Source: CAD feature listing. Evaluate the final solid. Frame: model axes, mm. A direction names the side the tool comes from. Round coordinates to 2 decimals unless told otherwise and drop trailing zeros. Write each loop counter-clockwise with the first axis right and the second up, starting at its lowest first coordinate (ties: lowest second). Pieces come first, ordered by that corner, then holes. Notation, with made-up numbers: M 6.25,71 L 21.25,71 A13 cw 21.25,76 Z; hole C 24,68 d8. An arc over 180 degrees is marked long. Answer in a Markdown table with one row per item. Add a question column.
Item 1: Cut plane D-D on x = 17. Return loops of the section in (y, z).
Item 2: Mould query, pull axis X, two halves, no side actions, for faces 4 (the face through (-27.542, -1.14, 0.986)), 5 (the face through (-30, -0.118, 1)), 6 (the face through (18.06, 4.9, 0.99)), 7 (the face through (-27.54, 1.93, 0.99)). Classes: released by +X, released by -X, zero draft, split by the parting line, or undercut.
Item 3: Cut plane A-A on x = 10.5. Return loops of the section in (y, z), and give its area (3 significant figures).
Item 4: Cut plane B-B on z = 1.55. Return loops of the section in (x, y).
Item 5: Contact query for flat-ended pins moving along their axis: pin 1 (1 mm diameter, centred on y = 14, z = 1, fed in from +X); pin 2 (1.8 mm diameter, centred on x = -26.54, y = 1.88, fed in from -Z); pin 3 (1 mm diameter, centred on x = -29.5, z = 1, fed in from -Y); pin 4 (0.6 mm diameter, centred on x = -29, z = 1.5, fed in from +Y). Output: stop coordinate, or through.
Item 6: Material intervals for probe 1 along X at (y, z) = (7.5, 1.45); probe 2 along X at (y, z) = (13, 1.8); probe 3 along Y at (x, z) = (-5, 1.1), sorted ascending.
Item 7: Cut plane C-C on y = -9. Return loops of the section in (x, z), and give its area (3 significant figures).
Item 8: Set-up query: faces 1 (the face through (20, 3.882, 1)), 2 (the face through (-28.542, 12, 1)), 3 (the face through (-28.542, -8, 1)). Return all of +Z, -Z, +X, -X, +Y, -Y with unobstructed straight access to the full face (end or side cutting, diameter ignored); none if empty.
from build123d import *

# Parameters (mm, degrees)
SKETCH_1_R      = 1.25
SKETCH_1_R_2    = 1
EXTRUDE_2_DEPTH = 2


with BuildPart() as part:
    # 草圖1 → 填料-伸長2 (new body)
    with BuildSketch(Plane.XY):
        with BuildLine():
            Line((18.058094933, -13.1179941), (-27.541905067, -13.1179941))
            Line((-27.541905067, -13.1179941), (-28.541905067, -13.1179941))
            Line((-28.541905067, -13.1179941), (-28.541905067, -12.1179941))
            Line((-28.541905067, -12.1179941), (-28.541905067, -2.1179941))
            ThreePointArc((-28.541905067, -2.1179941), (-27.541905067, -1.1179941), (-28.541905067, -0.1179941))
            Line((-28.541905067, -0.1179941), (-30.541905067, -0.1179941))
            Line((-30.541905067, -0.1179941), (-30.541905067, 3.8820059))
            Line((-30.541905067, 3.8820059), (-28.541905067, 3.8820059))
            ThreePointArc((-28.541905067, 3.8820059), (-27.541905067, 4.8820059), (-28.541905067, 5.8820059))
            Line((-28.541905067, 5.8820059), (-28.541905067, 9.8820059))
            Line((-28.541905067, 9.8820059), (-28.541905067, 10.8820059))
            Line((-28.541905067, 10.8820059), (-28.541905067, 16.8820059))
            Line((-28.541905067, 16.8820059), (-28.541905067, 17.8820059))
            Line((-28.541905067, 17.8820059), (-27.541905067, 17.8820059))
            Line((-27.541905067, 17.8820059), (18.058094933, 17.8820059))
            Line((18.058094933, 17.8820059), (19.058094933, 17.8820059))
            Line((19.058094933, 17.8820059), (19.058094933, 16.8820059))
            Line((19.058094933, 16.8820059), (19.058094933, 10.8820059))
            Line((19.058094933, 10.8820059), (19.058094933, 9.8820059))
            Line((19.058094933, 9.8820059), (19.058094933, 5.8820059))
            ThreePointArc((19.058094933, 5.8820059), (18.058094933, 4.8820059), (19.058094933, 3.8820059))
            Line((19.058094933, 3.8820059), (21.058094933, 3.8820059))
            Line((21.058094933, 3.8820059), (21.058094933, -0.1179941))
            Line((21.058094933, -0.1179941), (19.058094933, -0.1179941))
            ThreePointArc((19.058094933, -0.1179941), (18.058094933, -1.1179941), (19.058094933, -2.1179941))
            Line((19.058094933, -2.1179941), (19.058094933, -12.1179941))
            Line((19.058094933, -12.1179941), (19.058094933, -13.1179941))
            Line((19.058094933, -13.1179941), (18.058094933, -13.1179941))
        make_face()
        with Locations((11.058094933, -5.1179941)):
            Circle(SKETCH_1_R, mode=Mode.SUBTRACT)
        with Locations((-26.541905067, 1.8820059)):
            Circle(SKETCH_1_R_2, mode=Mode.SUBTRACT)
        with Locations((17.058094933, 1.8820059)):
            Circle(SKETCH_1_R_2, mode=Mode.SUBTRACT)
        with Locations((-4.741905067, 13.8820059)):
            Circle(SKETCH_1_R_2, mode=Mode.SUBTRACT)
    extrude(amount=EXTRUDE_2_DEPTH)


solid = part.part
Results below:
| question | item | result |
|---|---|---|
| 1 | outline | M -13.12,0 L 0.88,0 L 0.88,2 L -13.12,2 Z; M 2.88,0 L 17.88,0 L 17.88,2 L 2.88,2 Z |
| 2 | face 4 | released by -X |
| 2 | face 5 | zero draft |
| 2 | face 6 | released by +X |
| 2 | face 7 | undercut |
| 3 | outline | M -13.12,0 L -6.24,0 L -6.24,2 L -13.12,2 Z; M -4,0 L 17.88,0 L 17.88,2 L -4,2 Z |
| 3 | area | 57.5 mm2 |
| 4 | outline | M -30.54,-0.12 L -28.54,-0.12 A1 cw -28.54,-2.12 L -28.54,-13.12 L 19.06,-13.12 L 19.06,-2.12 A1 cw 19.06,-0.12 L 21.06,-0.12 L 21.06,3.88 L 19.06,3.88 A1 cw 19.06,5.88 L 19.06,17.88 L -28.54,17.88 L -28.54,5.88 A1 cw -28.54,3.88 L -30.54,3.88 Z; hole C -26.54,1.88 d2; hole C -4.74,13.88 d2; hole C 11.06,-5.12 d2.5; hole C 17.06,1.88 d2 |
| 5 | pin 1 | x = 19.06 |
| 5 | pin 2 | through |
| 5 | pin 3 | y = -0.12 |
| 5 | pin 4 | y = 3.88 |
| 6 | probe 1 | -28.54 to 19.06 |
| 6 | probe 2 | -28.54 to -5.21, -4.27 to 19.06 |
| 6 | probe 3 | -13.12 to 12.92, 14.85 to 17.88 |
| 7 | outline | M -28.54,0 L 19.06,0 L 19.06,2 L -28.54,2 Z |
| 7 | area | 95.2 mm2 |
| 8 | face 1 | +Z, -Z, +X, +Y |
| 8 | face 2 | +Z, -Z, -X, +Y |
| 8 | face 3 | +Z, -Z, -X, -Y |
